For this review, take the finished solid that the model builds, in its own axes (mm). Face numbers are marked on the shaded views. A direction names the side the tool comes from. Give positions to 0.01 mm unless a question says otherwise; leave off trailing zeros. Answer as CSV lines item,"result".
from build123d import *

# Parameters (mm, degrees)
SKETCH_2_W      = 0.546487167
SKETCH_2_H      = 4.918384508
EXTRUDE_1_DEPTH = 3.6
EXTRUDE_2_DEPTH = 11
EXTRUDE_START   = 0.5
EXTRUDE_4_DEPTH = 0.5
EXTRUDE_5_DEPTH = 11.5


with BuildPart() as part:
    # 扫描1: sweep along a curve in space
    with BuildLine() as sweep_1_path:
        Line((60, 6.926609333, 5.902285627), (60, 9.459381174, 30))
        ThreePointArc((54.097714373, 5.685898899, 0), (58.275153099, 6.306254116, 1.724846901), (60, 6.926609333, 5.902285627))
        Line((5.902285627, 0.620355217, 0), (54.097714373, 5.685898899, 0))
        ThreePointArc((0, -0.620355217, 5.902285627), (1.724846901, 0, 1.724846901), (5.902285627, 0.620355217, 0))
        Line((0, -0.620355217, 5.902285627), (0, -2.627605882, 25))
    # 草图1 → 扫描1 (sweep)
    with BuildSketch(Plane(origin=(60, 9.459381174, 30), x_dir=(1, 0, 0), z_dir=(0, 0.10452846326765572, 0.9945218953682732))):
        with BuildLine():
            Line((-6, 3.25), (-5.5, 3.25))
            ThreePointArc((-5.5, 3.25), (-4.621320344, 1.128679656), (-2.5, 0.25))
            Line((-2.5, 0.25), (2.5, 0.25))
            ThreePointArc((2.5, 0.25), (4.621320344, 1.128679656), (5.5, 3.25))
            ThreePointArc((5.5, 3.25), (5.42374237, 3.922109036), (5.198846296, 4.56004911))
            Line((5.198846296, 4.56004911), (5.745577195, 4.56004911))
            ThreePointArc((5.745577195, 4.56004911), (5.935805596, 3.917262998), (6, 3.25))
            ThreePointArc((6, 3.25), (4.974873734, 0.775126266), (2.5, -0.25))
            Line((2.5, -0.25), (-2.5, -0.25))
            ThreePointArc((-2.5, -0.25), (-4.974873734, 0.775126266), (-6, 3.25))
        make_face()
    sweep(path=sweep_1_path.line)

    # 草图2 → 凸台-拉伸1 (add)
    with BuildSketch(Plane(origin=(0, -2.627605882, 25), x_dir=(1, 0, 0), z_dir=(0, -0.1045284632676537, 0.9945218953682733))):
        with Locations((-6.423000936, 0.189458264)):
            Rectangle(SKETCH_2_W, SKETCH_2_H)
    extrude(amount=EXTRUDE_1_DEPTH)

    # 草图3 → 凸台-拉伸2 (add)
    with BuildSketch(Plane.ZY.offset(6.696244519)):
        Polygon((28.343027017, -5.261208499), (29.016349178, 1.145023935), (29.760098321, 1.06685275), (29.08677616, -5.339379684), align=None)
    extrude(amount=-EXTRUDE_2_DEPTH)

    # 草图5 → 凸台-拉伸4 (add)
    with BuildSketch(Plane(origin=(0, 3.222030449, 30.655571978), x_dir=(1, 0, 0), z_dir=(0, 0.10452846326765573, 0.9945218953682732)).offset(EXTRUDE_START)):
        with BuildLine():
            Line((65.745577195, 10.831756906), (54, 9.521707796))
            ThreePointArc((54, 9.521707796), (55.025126266, 7.046834062), (57.5, 6.021707796))
            Line((57.5, 6.021707796), (62.5, 6.021707796))
            ThreePointArc((62.5, 6.021707796), (64.974873734, 7.046834062), (66, 9.521707796))
            ThreePointArc((66, 9.521707796), (65.935805596, 10.188970794), (65.745577195, 10.831756906))
        make_face()
    extrude(amount=-EXTRUDE_4_DEPTH)

    # 草图6 → 凸台-拉伸5 (add)
    with BuildSketch(Plane(origin=(42.920636483, 14.309369815, 26.591437724), x_dir=(0, 0, 1), z_dir=(-0.9862492496089712, 0.16526468965190708, -2.582698329999371e-13))):
        with BuildLine():
            ThreePointArc((3.06884477, 2.502193657), (3.331726952, 2.738610574), (3.568143869, 2.475728392))
            ThreePointArc((3.568143869, 2.475728392), (2.699777506, 0.459022922), (0.729316838, -0.509711228))
            Line((0.729316838, -0.509711228), (-0.642859848, -0.651949655))
            ThreePointArc((-0.642859848, -0.651949655), (-2.66156717, -0.179875455), (-3.957168488, 1.438596209))
            ThreePointArc((-3.957168488, 1.438596209), (-3.805502668, 1.75796665), (-3.486132226, 1.606300829))
            ThreePointArc((-3.486132226, 1.606300829), (-2.093455907, 0.078991816), (-0.027928349, 0.002728684))
            Line((-0.027928349, 0.002728684), (0.142811981, -0.013953159))
            ThreePointArc((0.142811981, -0.013953159), (2.143390616, 0.618987912), (3.06884477, 2.502193657))
        make_face()
    extrude(amount=-EXTRUDE_5_DEPTH)


solid = part.part
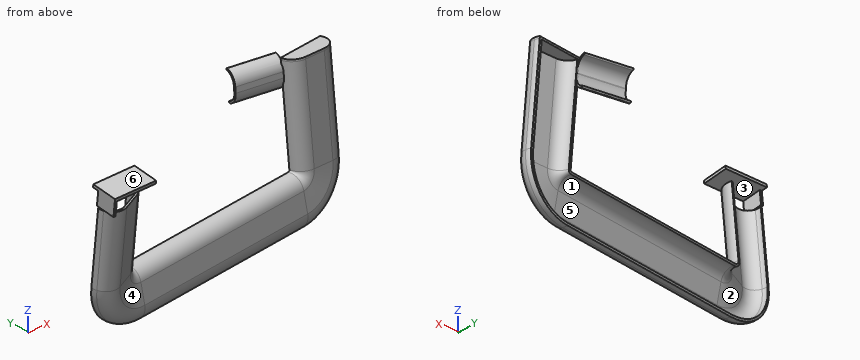
1) Insertion check: P1, Ø0.7, axis at y = -1, z = 29, coming from the +X side; P2, Ø1, axis at y = 8.5, z = 3, coming from the +X side; P3, Ø6, axis at x = 57.5, y = 8.5, coming from the -Z side. Each pin has a flat end and moves straight along its axis. Give the tip position at first contact, or say it passes through.
From the geometry:
P1,"stops at x = 4.3"
P2,"stops at x = 65.62"
P3,"stops at z = -6.6"
2) Wall thickness on line 1 (X direction, y = 10, z = 7); line 2 (X direction, y = -0.25, z = 11); line 3 (Z direction, x = 47.5, y = 14.5): over which ranges is each line inside the solid? List them lowest first. Write a range as from..to.
From the geometry:
line 1,"x = 54.01..54.52, 65.48..65.99"
line 2,"x = -6.94..-6.41, 1.42..2.63"
line 3,"z = 22.86..23.45, 29.05..29.67"
3) Machinability: for the marked faces 5 and 6, which of the approach directions +Z, -Z, +X, -X, +Y, -Y give a long, thin tool a straight path to every point of the face, cutting with its end or side? Answer none if there is none.
From the geometry:
face 5,"+Y"
face 6,"+Z, +X, -X, -Y"
4) Draft analysis for pull direction X (two halves, no side actions). For the marked faces 1, 2, 3 and 4, state which applies: pulls with the +X half, pulls with the -X half, needs draft (parallel to the pull), parting line crosses it, or undercut.
From the geometry:
face 1,"undercut"
face 2,"undercut"
face 3,"needs draft"
face 4,"pulls with the +X half"
